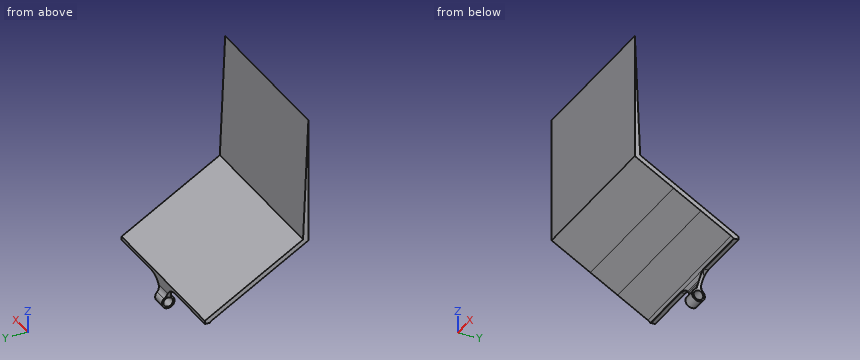
```python
from build123d import *

# Parameters (mm, degrees)
SKETCH1_R           = 3
BOSS_EXTRUDE1_DEPTH = 50
SKETCH2_W           = 49.237563161
SKETCH2_H           = 20.165956609
CUT_EXTRUDE1_DEPTH  = 35
FILLET1_R           = 10
FILLET3_START       = -50
FILLET3_DEPTH       = 100
FILLET3_START_2     = -14.0000001
FILLET3_2_DEPTH     = 28.0000001
FILLET3_START_3     = 5.029081153
FILLET3_3_DEPTH     = 7.627254367
FILLET4_R           = 5


with BuildPart() as part:
    # Sketch1 → Boss-Extrude1 (new, symmetric)
    with BuildSketch(Plane(origin=(0, 0, 0), x_dir=(0, 0, -1), z_dir=(1, 0, 0))):
        with BuildLine():
            Line((8.951712986, 8.463111178), (1.809964066, 8.463111178))
            Line((1.809964066, 8.463111178), (-10.541427431, -12.930126439))
            Line((-10.541427431, -12.930126439), (-20.432636562, -30.062203202))
            Line((-20.432636562, -30.062203202), (-34.461620266, -54.361115756))
            Line((-34.461620266, -54.361115756), (-113.02909109, -54.361115756))
            Line((-113.02909109, -54.361115756), (-36.018105083, -51.005100845))
            Line((-36.018105083, -51.005100845), (-0.492985983, 10.526210382))
            Line((-0.492985983, 10.526210382), (8.951712986, 10.526210382))
            ThreePointArc((8.951712986, 10.526210382), (16.816412899, 9.49466078), (8.951712986, 8.463111178))
        make_face()
        with Locations((12.816412899, 9.49466078)):
            Circle(SKETCH1_R, mode=Mode.SUBTRACT)
    extrude(amount=BOSS_EXTRUDE1_DEPTH, both=True)

    # Sketch2 → Cut-Extrude1 (cut, symmetric)
    with BuildSketch(Plane(origin=(0, -11.420787425, -0.571112862), x_dir=(1, 0, 0), z_dir=(0, 0.9987520183198841, 0.04994402769058576))):
        Polygon((-41.345711691, -80.976381383), (-37.345711691, -80.976381383), (-37.345711691, -96.642858944), (-33.68226718, -102.621642139), (-29.345711691, -96.642858944), (-29.345711691, -80.976381383), (-25.345711691, -80.976381383), (-25.345711691, -96.642858944), (-21.68226718, -102.621642139), (-17.345711691, -96.642858944), (-17.345711691, -80.976381383), (-13.345711691, -80.976381383), (-13.345711691, -96.642858944), (-9.68226718, -102.621642139), (-5.345711691, -96.642858944), (-5.345711691, -80.976381383), (-1.345711691, -80.976381383), (-1.345711691, -96.642858944), (2.31773282, -102.621642139), (6.654288309, -96.642858944), (6.654288309, -80.976381383), (10.654288309, -80.976381383), (10.654288309, -96.642858944), (14.31773282, -102.621642139), (18.654288309, -96.642858944), (18.654288309, -80.976381383), (22.654288309, -80.976381383), (22.654288309, -96.642858944), (26.31773282, -102.621642139), (30.654288309, -96.642858944), (30.654288309, -80.976381383), (34.654288309, -80.976381383), (34.654288309, -96.642858944), (38.31773282, -102.621642139), (42.654288309, -96.642858944), (42.654288309, -80.976381383), (46.654288309, -80.976381383), (46.654288309, -96.642858944), (50.31773282, -102.621642139), (54.654288309, -96.642858944), (54.654288309, -80.976381383), (58.654288309, -80.976381383), (58.654288309, -96.642858944), (58.654288309, -117.647520094), (-58.342792285, -117.647520094), (-58.342792285, -96.642858944), (-49.345711691, -96.642858944), (-45.68226718, -102.621642139), (-41.345711691, -96.642858944), align=None)
        with Locations((-28.618781581, 12.150846953)):
            Rectangle(SKETCH2_W, SKETCH2_H)
        with Locations((28.618781581, 12.150846953)):
            Rectangle(SKETCH2_W, SKETCH2_H)
    extrude(amount=CUT_EXTRUDE1_DEPTH, both=True, mode=Mode.SUBTRACT)

    # Fillet1
    # the kernel refuses this fillet: 10 mm, written as the material it adds along each edge
    with BuildSketch(Plane(origin=(-4, 35.49501084, -0.295473589), x_dir=(0, 0.049944027690585764, -0.9987520183198841), z_dir=(0, -0.9987520183198841, -0.04994402769058576))) as fillet1_piece_1_section:
        with BuildLine():
            CenterArc((FILLET1_R, -FILLET1_R), FILLET1_R, 90, 90)
            Line((0, -FILLET1_R), (0, 0))
            Line((0, 0), (FILLET1_R, 0))
        make_face()
    fillet1_piece_1 = extrude(amount=52.325377672, mode=Mode.PRIVATE)
    fillet1_piece_1 = split(fillet1_piece_1, bisect_by=Plane(origin=(-4, 8.463111178, -0.295473589), z_dir=(0, 1, 0)), keep=Keep.TOP, mode=Mode.PRIVATE)
    fillet1_piece_1 = split(fillet1_piece_1, bisect_by=Plane(origin=(-4, 10.526210382, -0.295473589), z_dir=(0, -1, 0)), keep=Keep.TOP, mode=Mode.PRIVATE)
    fillet1_piece_1 = fillet1_piece_1 - Plane(origin=(-4, 9.49466078, -12.816412899), x_dir=(0, 0, -1), z_dir=(-1, 0, 0)) * Cylinder(3, 145, mode=Mode.PRIVATE)
    add(fillet1_piece_1)
    with BuildSketch(Plane(origin=(-4, 35.49501084, -0.295473589), x_dir=(0, 0.049944027690585764, -0.9987520183198841), z_dir=(0, -0.9987520183198841, -0.04994402769058576))) as fillet1_piece_2_section:
        with BuildLine():
            CenterArc((FILLET1_R, -FILLET1_R), FILLET1_R, 90, 90)
            Line((0, -FILLET1_R), (0, 0))
            Line((0, 0), (FILLET1_R, 0))
        make_face()
    fillet1_piece_2 = extrude(amount=52.325377672, mode=Mode.PRIVATE)
    fillet1_piece_2 = split(fillet1_piece_2, bisect_by=Plane(origin=(-4, 28.081242311, -13.136497357), z_dir=(0, 0.4999999999999977, 0.8660254037844399)), keep=Keep.TOP, mode=Mode.PRIVATE)
    fillet1_piece_2 = split(fillet1_piece_2, bisect_by=Plane(origin=(-4, 10.526210382, -0.295473589), z_dir=(0, -1, 0)), keep=Keep.TOP, mode=Mode.PRIVATE)
    add(fillet1_piece_2)
    with BuildSketch(Plane(origin=(-4, 35.49501084, -0.295473589), x_dir=(0, 0.049944027690585764, -0.9987520183198841), z_dir=(0, -0.9987520183198841, -0.04994402769058576))) as fillet1_piece_3_section:
        with BuildLine():
            CenterArc((FILLET1_R, -FILLET1_R), FILLET1_R, 90, 90)
            Line((0, -FILLET1_R), (0, 0))
            Line((0, 0), (FILLET1_R, 0))
        make_face()
    fillet1_piece_3 = extrude(amount=52.325377672, mode=Mode.PRIVATE)
    fillet1_piece_3 = fillet1_piece_3 & Plane(origin=(-4, 9.49466078, -12.816412899), x_dir=(0, 0.2578874004491323, 0.9661749782982318), z_dir=(1, 0, 0)) * Cylinder(4, 145, mode=Mode.PRIVATE)
    fillet1_piece_3 = fillet1_piece_3 - Plane(origin=(-4, 9.49466078, -12.816412899), x_dir=(0, 0, -1), z_dir=(-1, 0, 0)) * Cylinder(3, 145, mode=Mode.PRIVATE)
    add(fillet1_piece_3)
    with BuildSketch(Plane(origin=(4, -16.76506572, -2.908813701), x_dir=(0, 0.049944027690585764, -0.9987520183198841), z_dir=(0, 0.9987520183198841, 0.04994402769058576))) as fillet1_piece_4_section:
        with BuildLine():
            CenterArc((FILLET1_R, -FILLET1_R), FILLET1_R, 90, 90)
            Line((0, -FILLET1_R), (0, 0))
            Line((0, 0), (FILLET1_R, 0))
        make_face()
    fillet1_piece_4 = extrude(amount=52.325377672, mode=Mode.PRIVATE)
    fillet1_piece_4 = split(fillet1_piece_4, bisect_by=Plane(origin=(4, -9.982205646, 8.839444568), z_dir=(0, 0.4999999999999977, 0.8660254037844399)), keep=Keep.TOP, mode=Mode.PRIVATE)
    fillet1_piece_4 = split(fillet1_piece_4, bisect_by=Plane(origin=(4, 10.526210382, -2.908813701), z_dir=(0, -1, 0)), keep=Keep.TOP, mode=Mode.PRIVATE)
    add(fillet1_piece_4)
    with BuildSketch(Plane(origin=(4, -16.76506572, -2.908813701), x_dir=(0, 0.049944027690585764, -0.9987520183198841), z_dir=(0, 0.9987520183198841, 0.04994402769058576))) as fillet1_piece_5_section:
        with BuildLine():
            CenterArc((FILLET1_R, -FILLET1_R), FILLET1_R, 90, 90)
            Line((0, -FILLET1_R), (0, 0))
            Line((0, 0), (FILLET1_R, 0))
        make_face()
    fillet1_piece_5 = extrude(amount=52.325377672, mode=Mode.PRIVATE)
    fillet1_piece_5 = split(fillet1_piece_5, bisect_by=Plane(origin=(4, 8.463111178, -2.908813701), z_dir=(0, 1, 0)), keep=Keep.TOP, mode=Mode.PRIVATE)
    fillet1_piece_5 = split(fillet1_piece_5, bisect_by=Plane(origin=(4, 10.526210382, -2.908813701), z_dir=(0, -1, 0)), keep=Keep.TOP, mode=Mode.PRIVATE)
    fillet1_piece_5 = fillet1_piece_5 - Plane(origin=(4, 9.49466078, -12.816412899), x_dir=(0, 0, -1), z_dir=(-1, 0, 0)) * Cylinder(3, 145, mode=Mode.PRIVATE)
    add(fillet1_piece_5)
    with BuildSketch(Plane(origin=(4, -16.76506572, -2.908813701), x_dir=(0, 0.049944027690585764, -0.9987520183198841), z_dir=(0, 0.9987520183198841, 0.04994402769058576))) as fillet1_piece_6_section:
        with BuildLine():
            CenterArc((FILLET1_R, -FILLET1_R), FILLET1_R, 90, 90)
            Line((0, -FILLET1_R), (0, 0))
            Line((0, 0), (FILLET1_R, 0))
        make_face()
    fillet1_piece_6 = extrude(amount=52.325377672, mode=Mode.PRIVATE)
    fillet1_piece_6 = fillet1_piece_6 & Plane(origin=(4, 9.49466078, -12.816412899), x_dir=(0, 0.2578874004491323, 0.9661749782982318), z_dir=(1, 0, 0)) * Cylinder(4, 145, mode=Mode.PRIVATE)
    fillet1_piece_6 = fillet1_piece_6 - Plane(origin=(4, 9.49466078, -12.816412899), x_dir=(0, 0, -1), z_dir=(-1, 0, 0)) * Cylinder(3, 145, mode=Mode.PRIVATE)
    add(fillet1_piece_6)

    # Fillet3: read off the stored shape, not the designer's step
    # Fillet3 outline → Fillet3 (add)
    with BuildSketch(Plane.YZ.offset(FILLET3_START)):
        with BuildLine():
            Line((7.463496818, -1.697229668), (8.203734738, -1.660213009))
            Line((8.203734738, -1.660213009), (5.963111178, -0.366588393))
            ThreePointArc((5.963111178, -0.366588393), (6.780701406, -0.955914016), (7.463496818, -1.697229668))
        make_face()
    extrude(amount=FILLET3_DEPTH)

    # Fillet3 2 outline → Fillet3 2 (add)
    with BuildSketch(Plane.YZ.offset(FILLET3_START_2)):
        with BuildLine():
            Line((8.463111178, -1.809964066), (8.203734738, -1.660213009))
            Line((8.203734738, -1.660213009), (7.463496818, -1.697229668))
            ThreePointArc((7.463496818, -1.697229668), (8.206629292, -3.115881487), (8.463111178, -4.696715412))
            Line((8.463111178, -4.696715412), (8.463111178, -1.809964066))
        make_face()
    extrude(amount=FILLET3_2_DEPTH)

    # Fillet3 3 outline → Fillet3 3 (cut)
    with BuildSketch(Plane(origin=(0, 0, 0), x_dir=(1, 0, 0), z_dir=(0, 0.998752018319884, 0.0499440276905858)).offset(FILLET3_START_3)):
        with BuildLine():
            ThreePointArc((-14, 2.067868648), (-9.034050266, 3.38804473), (-5.379286145, 7))
            Line((-5.379286145, 7), (-14.0000001, 7))
            Line((-14.0000001, 7), (-14, 2.067868648))
        make_face()
        with BuildLine():
            Line((14, 7), (5.379286145, 7))
            ThreePointArc((5.379286145, 7), (9.034050266, 3.38804473), (14, 2.067868648))
            Line((14, 2.067868648), (14, 7))
        make_face()
    extrude(amount=FILLET3_3_DEPTH, mode=Mode.SUBTRACT)

    # Fillet4
    # the kernel refuses this fillet: 5 mm, written as the material it adds along each edge
    with BuildSketch(Plane(origin=(-11.410578331, 8.463111178, -8.951712972), x_dir=(-4.3911864757766885e-10, -0.8787125753545649, -0.47735124375426957), z_dir=(1.0, 9.37113186758836e-13, -9.216318308073321e-10))) as fillet4_piece_1_section:
        with BuildLine():
            CenterArc((3.049747005, -4.860464878), FILLET4_R, 103.567804979, 47.919645029)
            Line((-1.343815871, -2.473708659), (0, 0))
            ThreePointArc((0, 0), (0.938383697, -0.111628098), (1.876767394, 0))
        make_face()
    fillet4_piece_1 = extrude(amount=15.410578331, mode=Mode.PRIVATE)
    fillet4_piece_1 = fillet4_piece_1 - Plane(origin=(-14, 8.598192062, -11.652983015), x_dir=(0, 0.04994402769099318, -0.9987520183198637), z_dir=(0, 0.9987520183198637, 0.04994402769099318)) * Cylinder(10, 41, mode=Mode.PRIVATE)
    add(fillet4_piece_1)
    with BuildSketch(Plane(origin=(-11.382224103, 10.526210382, -8.951712986), x_dir=(4.174135827959178e-15, 0.8787125762173496, -0.47735124216604746), z_dir=(1, 0, 0))) as fillet4_piece_2_section:
        with BuildLine():
            CenterArc((3.049747012, 4.860464876), FILLET4_R, 208.512549888, 47.919645029)
            Line((-1.343815869, 2.473708665), (0, 0))
            ThreePointArc((0, 0), (0.938383696, 0.111628099), (1.876767392, 0))
        make_face()
    fillet4_piece_2 = extrude(amount=22.764448206, mode=Mode.PRIVATE)
    fillet4_piece_2 = fillet4_piece_2 - Plane(origin=(14, 10.656145058, -11.550072123), x_dir=(0, 0.04994402769099318, -0.9987520183198637), z_dir=(0, -0.9987520183198637, -0.04994402769099318)) * Cylinder(10, 56, mode=Mode.PRIVATE)
    fillet4_piece_2 = fillet4_piece_2 - Plane(origin=(-14, 10.656145058, -11.550072123), x_dir=(0, 0.04994402769099318, -0.9987520183198637), z_dir=(0, 0.9987520183198637, 0.04994402769099318)) * Cylinder(10, 56, mode=Mode.PRIVATE)
    add(fillet4_piece_2)
    with BuildSketch(Plane(origin=(4, 8.463111178, -8.951712986), x_dir=(0, -0.8787125762172517, -0.4773512421662278), z_dir=(1, 0, 0))) as fillet4_piece_3_section:
        with BuildLine():
            CenterArc((3.049747012, -4.860464876), FILLET4_R, 103.567805083, 47.919645029)
            Line((-1.343815869, -2.473708665), (0, 0))
            ThreePointArc((0, 0), (0.938383696, -0.111628099), (1.876767392, 0))
        make_face()
    fillet4_piece_3 = extrude(amount=7.41057834, mode=Mode.PRIVATE)
    fillet4_piece_3 = fillet4_piece_3 - Plane(origin=(14, 8.598192062, -11.652983015), x_dir=(0, 0.04994402769099318, -0.9987520183198637), z_dir=(0, -0.9987520183198637, -0.04994402769099318)) * Cylinder(10, 25, mode=Mode.PRIVATE)
    add(fillet4_piece_3)


solid = part.part
```
Input: part model. Units: mm. Frame: model coordinates. Give positions to 0.01 mm unless a question says otherwise; leave off trailing zeros. Loops run counter-clockwise (first coordinate to the right, second up) from the corner with the lowest first, then second, coordinate; pieces in that order, holes last.
1) Section query A-A on x = 28.5. Return the cut outline in (y, z), and give its area (3 significant figures).
A:
outline: (-54.36, 34.46) - (5.96, -0.37) arc R5 cw to (7.46, -1.7) - (10.53, -1.54) - (10.53, 0.49) - (-51.01, 36.02) - (-54.36, 113.03) - close
area: 351 mm2
2) Section query C-C on z = 64. Return the cut outline in (x, y).
A:
outline: (-50, -54.36) - (50, -54.36) - (50, -52.22) - (-50, -52.22) - close
3) Contact query for flat-ended pins moving along their axis: pin 1 (1.5 mm diameter, centred on x = -26, z = 11, fed in from +Y); pin 2 (7 mm diameter, centred on y = 9.49, z = -12.82, fed in from -X); pin 3 (2 mm diameter, centred on x = 2, z = -2.5, fed in from +Y); pin 4 (2.5 mm diameter, centred on y = 8.5, z = -13, fed in from +X). Output: stop coordinate, or through.
A:
pin 1: stops at y = -6.37
pin 2: stops at x = -4.27
pin 3: stops at y = 10.53
pin 4: passes through
4) Line query: L1, parallel to Z at x = 29, y = -28; L2, parallel to Y at x = 9, z = 29.5; L3, parallel to Y at x = -36, z = 62.5. Output: solid intervals per line, ascending.
A:
L1: z = 19.24 to 22.74
L2: y = -45.77 to -39.72
L3: y = -54.36 to -52.16
5) Section query B-B on y = -2. Return the cut outline in (x, z) (3 decimals), and give its area (3 significant figures).
A:
outline: (-50, 4.231) - (50, 4.231) - (50, 7.725) - (-50, 7.725) - close
area: 349 mm2
